```python
from build123d import *

# Parameters (mm, degrees)
SKETCH005_R          = 35
SKETCH005_R_2        = 25
PAD_DEPTH            = 10
SKETCH006_R          = 32.2
SKETCH006_R_2        = 25
PAD001_DEPTH         = 3
SKETCH_R             = 35
SKETCH_R_2           = 28
PAD002_DEPTH         = 17
SKETCH004_R          = 1.5
POCKET_DEPTH         = 20
SKETCH003_R          = 1.5
POCKET001_DEPTH      = 8.5
POCKET001_DEPTH_BACK = 100
PAD003_DEPTH         = 0.01
PAD003_DEPTH_BACK    = 15
POLARPATTERN_COUNT   = 4


with BuildPart() as part:
    # Sketch005 → Pad (new body)
    with BuildSketch(Plane.XY.offset(-1.5)):
        Circle(SKETCH005_R)
        Circle(SKETCH005_R_2, mode=Mode.SUBTRACT)
    extrude(amount=-PAD_DEPTH)

    # Sketch006 → Pad001 (join)
    with BuildSketch(Plane.XY.offset(-1.5)):
        Circle(SKETCH006_R)
        Circle(SKETCH006_R_2, mode=Mode.SUBTRACT)
    extrude(amount=PAD001_DEPTH)

    # Sketch → Pad002 (join)
    with BuildSketch(Plane.XY.offset(1.5)):
        Circle(SKETCH_R)
        Circle(SKETCH_R_2, mode=Mode.SUBTRACT)
    extrude(amount=PAD002_DEPTH)

    # Sketch004 → Pocket (cut)
    with BuildSketch(Plane(origin=(28, 0, 0), x_dir=(1, 0, 0), z_dir=(0, 0, 1))):
        Circle(SKETCH004_R)
    extrude(amount=POCKET_DEPTH, mode=Mode.SUBTRACT)

    # Sketch003 → Pocket001 (cut, two sides)
    with BuildSketch(Plane(origin=(35, 0, 0), x_dir=(0, 0.939693, 0.34202), z_dir=(1, 0, 0))) as pocket001_sk:
        Circle(SKETCH003_R)
    extrude(amount=-POCKET001_DEPTH, mode=Mode.SUBTRACT)
    extrude(pocket001_sk.sketch, amount=POCKET001_DEPTH_BACK, mode=Mode.SUBTRACT)

    # Sketch002 → Pad003 (join, two sides)
    with BuildSketch(Plane.XY.offset(-1.5)) as pad003_sk:
        with BuildLine():
            ThreePointArc((-34.997021, 0.456663), (-33.922719, -8.616793), (-30.53664, -17.103029))
            Line((-30.53664, -17.103029), (-21.762611, -12.504957))
            ThreePointArc((-25.093421, 0), (-24.251171, -6.471733), (-21.762611, -12.504957))
            Line((-34.997021, 0.456663), (-25.093421, 0))
        make_face()
    pad003 = extrude(amount=PAD003_DEPTH) + extrude(pad003_sk.sketch, amount=-PAD003_DEPTH_BACK)

    # PolarPattern: Pad003 ×4 about axis
    polarpattern_axis = Axis((0, 0, -1.5), (0, 0, 1))
    for i in range(1, POLARPATTERN_COUNT):
        add(pad003.rotate(polarpattern_axis, i * 360 / POLARPATTERN_COUNT))


solid = part.part
```
Design review of the part built by this model. Coordinates are the model's own, in mm. A direction names the side the tool comes from. Round coordinates to 2 decimals unless told otherwise and drop trailing zeros. Order: outer loops, then holes, each group sorted by start corner. A loop starts at its lowest first (then second) coordinate and runs counter-clockwise, first axis right, second up. Notation, with made-up numbers: (4.25, 33.25) - (27.25, 33.25) arc R29 ccw to (27.25, 63.25) - close; hole circle Ø11 at (30, 4.5). An arc over 180 degrees is marked (long way). Return JSON: item names as keys, results as strings.
Q1. Consider section D-D on x = 24. Write out the cut boundary in (y, z).
Computed values:
{"outline": "(-25.48, -11.5) - (-7, -11.5) - (-7, 1.5) - (-14.42, 1.5) - (-14.42, 18.5) - (-25.48, 18.5) - (-25.48, 1.5) - (-21.47, 1.5) - (-21.47, -1.5) - (-25.48, -1.5) - close; (7, -11.5) - (7.35, -11.5) - (7.35, -16.5) - (13.68, -16.5) - (13.68, -11.5) - (25.48, -11.5) - (25.48, -1.5) - (21.47, -1.5) - (21.47, 1.5) - (25.48, 1.5) - (25.48, 18.5) - (14.42, 18.5) - (14.42, 1.5) - (7, 1.5) - close"}
Q2. Consider section A-A on x = -19.5. Write out the cut boundary in (y, z), plus the area to 3 significant figures.
Computed values:
{"outline": "(-29.06, -11.5) - (-15.64, -11.5) - (-15.64, 1.5) - (-20.09, 1.5) - (-20.09, 18.5) - (-29.06, 18.5) - (-29.06, 1.5) - (-25.62, 1.5) - (-25.62, -1.5) - (-29.06, -1.5) - close; (15.64, -11.5) - (29.06, -11.5) - (29.06, -1.5) - (25.62, -1.5) - (25.62, 1.5) - (29.06, 1.5) - (29.06, 18.5) - (20.09, 18.5) - (20.09, 1.5) - (15.64, 1.5) - close", "area": "633 mm2"}
Q3. Wall thickness on L1, parallel to Y at x = 0, z = 9.5; L2, parallel to Y at x = 0, z = -7; L3, parallel to Z at x = -21.5, y = -19.5: over which ranges is each line inside the solid? List them lowest first. Write a range as [from, to].
Computed values:
{"L1": "y = [-35, -28], [28, 35]", "L2": "y = [-35, -25], [25, 35]", "L3": "z = [-11.5, 18.5]"}
Q4. The part is to be moulded in two halves that separate along X. For faces 4 (the flat face through (-30.11, 0.23, -13.96)), 5 (the flat face through (-17, 19, 1.5)), 6 (the flat face through (0.23, 30.11, -14.04)), 7 (the flat face through (8, -32, -1.49)), say which applies: pulls with the +X half, pulls with the -X half, needs draft (parallel to the pull), parting line crosses it, or undercut.
Computed values:
{"face 4": "undercut", "face 5": "undercut", "face 6": "pulls with the +X half", "face 7": "needs draft"}
Q5. Consider section C-C on z = -10. Write out the cut boundary in (x, y), plus the area to 3 significant figures.
Computed values:
{"outline": "circle Ø70 at (0, 0); hole circle Ø50 at (0, 0)", "area": "1,880 mm2"}
Q6. Consider section B-B on y = 5.5. Write out the cut boundary in (x, z).
Computed values:
{"outline": "(-34.57, -11.5) - (-24.39, -11.5) - (-24.39, 1.5) - (-27.45, 1.5) - (-27.45, 18.5) - (-34.57, 18.5) - (-34.57, 1.5) - (-31.73, 1.5) - (-31.73, -1.5) - (-34.57, -1.5) - close; (24.39, -11.5) - (24.49, -11.5) - (24.49, -16.5) - (34.57, -16.5) - (34.57, -1.49) - (31.73, -1.49) - (31.73, 1.5) - (34.57, 1.5) - (34.57, 18.5) - (27.45, 18.5) - (27.45, 1.5) - (24.39, 1.5) - close"}
Q7. Machinability: for faces 1 (the flat face through (-14.836, 26.211, -14.035)), 2 (the flat face through (30.11, -0.23, -14.04)), 3 (the cylindrical face through (30.023, 0.602, -1.374)), which of the approach directions +Z, -Z, +X, -X, +Y, -Y give a long, thin tool a straight path to every point of the face, cutting with its end or side? Answer none if there is none.
Computed values:
{"face 1": "-Z, -X, -Y", "face 2": "-Z, -Y", "face 3": "+X"}
Q8. For pin 1 Ø12 at (y, z) = (-25, 0) entering from -X; pin 2 Ø15.5 at (x, y) = (-21, -30) entering from +Z; pin 3 Ø6 at (x, z) = (-18, -3.5) entering from +Y; pin 4 Ø2.5 at (y, z) = (0, 0) entering from +X, all flat-tipped, find the tip position at first contact; note any pin that passes through.
Computed values:
{"pin 1": "stops at x = -29.27", "pin 2": "stops at z = 18.5", "pin 3": "stops at y = 31.62", "pin 4": "stops at x = 26.5"}
